Input: part model. Units: mm. Frame: model coordinates. Give positions to 0.01 mm unless a question says otherwise; leave off trailing zeros. Loops run counter-clockwise (first coordinate to the right, second up) from the corner with the lowest first, then second, coordinate; pieces in that order, holes last.
from build123d import *

# Parameters (mm, degrees)
F1_DEPTH = 3.175


# Not quite as in the source:
# - a length typed as a fraction of an inch, garbled in the dataset ("3 / 203.2 mm" for 3/8 in), is restored


with BuildPart() as f1:
    # F0 (on Front) → F1 (new body)
    with BuildSketch(Plane.XZ):
        Polygon((-193.675, 0), (0, 0), (0, 139.7), (-317.1003863096, 139.7), (-325.2376931548, 131.5626931548), align=None)
        Polygon((0, 139.7), (0, 0), (193.675, 0), (325.2376931548, 131.5626931548), (317.1003863096, 139.7), align=None)
    extrude(amount=F1_DEPTH)


solid = f1.part
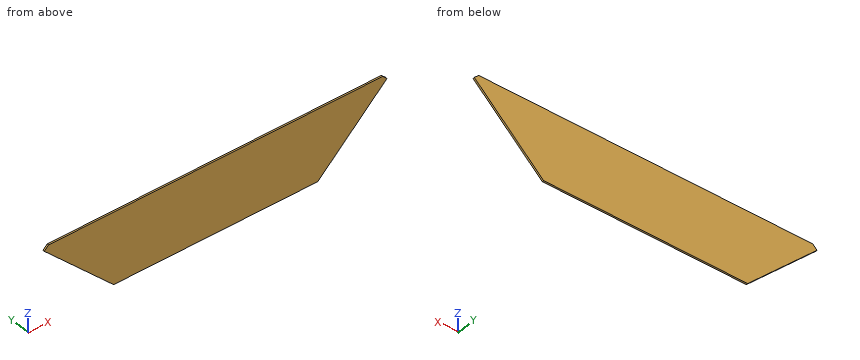
(1) Ray query, probe 1 along X at (y, z) = (-2.2, 92.5) (3 decimals); probe 2 along X at (y, z) = (-2.85, 53) (3 decimals); probe 3 along Z at (x, y) = (201.5, -0.4) (3 decimals). Return the intervals inside material, ascending.
Values follow:
probe 1: x = -286.175 to 286.175
probe 2: x = -246.675 to 246.675
probe 3: z = 7.825 to 139.7
(2) Pin query (flat end, axial travel): pin 1 Ø1.5 at (y, z) = (-0.5, 119) entering from +X (3 decimals). Return the tip coordinate at first contact, or that it passes through.
Values follow:
pin 1: stops at x = 313.425
(3) Cut plane B-B (z = 15.5). Return the cut outline in (x, y) (3 decimals).
Values follow:
outline: (-209.175, -3.175) - (209.175, -3.175) - (209.175, 0) - (-209.175, 0) - close
(4) Cut plane C-C (x = 271.5). Return the cut outline in (y, z) (3 decimals), and give its area (3 significant figures).
Values follow:
outline: (-3.175, 77.825) - (0, 77.825) - (0, 139.7) - (-3.175, 139.7) - close
area: 196 mm2
(5) Cut plane A-A (y = -2.65). Return the cut outline in (x, z) (3 decimals), and give its area (3 significant figures).
Values follow:
outline: (-325.238, 131.563) - (-193.675, 0) - (193.675, 0) - (325.238, 131.563) - (317.1, 139.7) - (-317.1, 139.7) - close
area: 73,500 mm2
